```python
from build123d import *

# Parameters (mm, degrees)
BOSS_EXTRU_1_DEPTH      = 5
ESQUISSE2_R             = 1.6
ENL_V_MAT_EXTRU_1_DEPTH = 209.56953277


with BuildPart() as part:
    # Esquisse1 → Boss.-Extru.1 (new body)
    with BuildSketch(Plane(origin=(0, 0, 0), x_dir=(1, 0, 0), z_dir=(0, 1, 0))):
        with BuildLine():
            Line((-50.5, 31.2), (-35.5, 31.2))
            Line((-35.5, 31.2), (-35.5, 21.2))
            Line((-35.5, 21.2), (35.5, 21.2))
            Line((35.5, 21.2), (35.5, 31.2))
            Line((35.5, 31.2), (50.5, 31.2))
            Line((50.5, 31.2), (50.5, -21.2))
            Line((50.5, -21.2), (123.5, -21.2))
            Line((123.5, -21.2), (123.5, -168))
            Line((123.5, -168), (113.5, -168))
            Line((113.5, -168), (13.488258165, -134.084795517))
            ThreePointArc((13.488258165, -134.084795517), (0, -131.86), (-13.488258165, -134.084795517))
            Line((-13.488258165, -134.084795517), (-113.5, -168))
            Line((-113.5, -168), (-123.5, -168))
            Line((-123.5, -168), (-123.5, -21.2))
            Line((-123.5, -21.2), (-50.5, -21.2))
            Line((-50.5, -21.2), (-50.5, 31.2))
        make_face()
    extrude(amount=BOSS_EXTRU_1_DEPTH)

    # Esquisse2 → Enlèv. mat.-Extru.1 (cut, through all)
    with BuildSketch(Plane.XZ):
        with Locations(Location((-118.5, 163, 0), (0, 0, 270))):
            Circle(ESQUISSE2_R)
        with Locations(Location((118.5, 163, 0), (0, 0, 270))):
            Circle(ESQUISSE2_R)
        with Locations(Location((118.5, 26.2, 0), (0, 0, 270))):
            Circle(ESQUISSE2_R)
        with Locations(Location((-118.5, 26.2, 0), (0, 0, 270))):
            Circle(ESQUISSE2_R)
        with Locations(Location((43, -26.2, 0), (0, 0, 270))):
            Circle(ESQUISSE2_R)
        with Locations(Location((-43, -26.2, 0), (0, 0, 270))):
            Circle(ESQUISSE2_R)
        with Locations(Location((20.859650045, 38.859650045, 0), (0, 0, 270))):
            Circle(ESQUISSE2_R)
        with Locations(Location((-20.859650045, 38.859650045, 0), (0, 0, 270))):
            Circle(ESQUISSE2_R)
        with Locations(Location((-20.859650045, -2.859650045, 0), (0, 0, 270))):
            Circle(ESQUISSE2_R)
        with Locations(Location((20.859650045, -2.859650045, 0), (0, 0, 270))):
            Circle(ESQUISSE2_R)
        with Locations(Location((0, 123.86, 0), (0, 0, 270))):
            Circle(ESQUISSE2_R)
    extrude(amount=-ENL_V_MAT_EXTRU_1_DEPTH, mode=Mode.SUBTRACT)


solid = part.part
```
Build history of the part. All positions in model axes, mm. A direction names the side the tool comes from. Give positions to 0.01 mm unless a question says otherwise; leave off trailing zeros. Loops run counter-clockwise (first coordinate to the right, second up) from the corner with the lowest first, then second, coordinate; pieces in that order, holes last. Notation, with made-up numbers: (49, -40) -> (77, -40) arc R16 cw to (77, -24) -> close; hole circle Ø4 at (82.25, 75.5). An arc over 180 degrees is marked (long way). One line per question, with ' | ' between items.
Q1. Drill centre lines: line 1 along Z through (x, y) = (-118.5, 2.15); line 2 along X through (y, z) = (2.6, -26.2); line 3 along X through (y, z) = (3.35, -19). Where is each one in solid material? Low to high. Write a range as [from, to].
Filled sheet:
line 1: z = [21.2, 24.6], [27.8, 161.4], [164.6, 168] | line 2: x = [-50.5, -44.6], [-41.4, -35.5], [35.5, 41.4], [44.6, 50.5] | line 3: x = [-50.5, 50.5]
Q2. Cut at B-B, the plane x = 10. Write the cut outline in (y, z), plus the area to 3 significant figures.
Filled sheet:
outline: (0, -21.2) -> (5, -21.2) -> (5, 133.07) -> (0, 133.07) -> close | area: 771 mm²
Q3. Drop flat-ended pins along their axis: pin 1 (2.5 mm diameter, centred on x = -20.86, z = -2.86, fed in from +Y); pin 2 (2.5 mm diameter, centred on y = 3, z = 8, fed in from +X); pin 3 (1.5 mm diameter, centred on x = -98, y = 1.5, fed in from -Z); pin 4 (1.5 mm diameter, centred on y = 1.5, z = -24.5, fed in from -X). Give the stop position or say it passes through.
Filled sheet:
pin 1: passes through | pin 2: stops at x = 50.5 | pin 3: stops at z = 21.2 | pin 4: stops at x = -50.5
Q4. Tool access for faces 1 (the flat face through (64.19, 2.46, 151.28)), 2 (the flat face through (86, 2, 21.2)), 3 (the flat face through (35.5, 2, -26)): list every direction of +Z, -Z, +X, -X, +Y, -Y with a clear straight run to the whole face (end or side of a thin tool).
Filled sheet:
face 1: +Z, +Y, -Y | face 2: -Z, +X, +Y, -Y | face 3: -Z, +Y, -Y
Q5. Cut at C-C, the plane x = -26. Write the cut outline in (y, z), plus the area to 3 significant figures.
Filled sheet:
outline: (0, -21.2) -> (5, -21.2) -> (5, 138.33) -> (0, 138.33) -> close | area: 798 mm²
Q6. Cut at A-A, the plane y = 1.1. Count the separate pieces of the cut face and the enclosed holes in it, plus the area to 3 significant figures.
Filled sheet:
separate pieces: 1 | enclosed holes: 11 | area: 36,400 mm²
